from build123d import *

# Parameters (mm, degrees)
SKETCH1_R           = 1.3
SKETCH1_W           = 14
SKETCH1_H           = 14
BOSS_EXTRUDE1_DEPTH = 1


with BuildPart() as part:
    # Sketch1 → Boss-Extrude1 (new body)
    with BuildSketch(Plane(origin=(0, 0, 0), x_dir=(1, 0, 0), z_dir=(0, 1, 0))):
        with BuildLine():
            Line((27.6, 52), (-27.6, 52))
            ThreePointArc((-27.6, 52), (-28.660660172, 51.560660172), (-29.1, 50.5))
            Line((-29.1, 50.5), (-29.1, -50.5))
            ThreePointArc((-29.1, -50.5), (-28.660660172, -51.560660172), (-27.6, -52))
            Line((-27.6, -52), (27.6, -52))
            ThreePointArc((27.6, -52), (28.660660172, -51.560660172), (29.1, -50.5))
            Line((29.1, -50.5), (29.1, 50.5))
            ThreePointArc((29.1, 50.5), (28.660660172, 51.560660172), (27.6, 52))
        make_face()
        with Locations(Location((-9.525, -32.95, 0), (0, 0, 270))):
            Circle(SKETCH1_R, mode=Mode.SUBTRACT)
        with Locations(Location((9.525, -32.95, 0), (0, 0, 270))):
            Circle(SKETCH1_R, mode=Mode.SUBTRACT)
        with Locations(Location((9.525, 24.2, 0), (0, 0, 270))):
            Circle(SKETCH1_R, mode=Mode.SUBTRACT)
        with Locations(Location((-9.525, 24.2, 0), (0, 0, 270))):
            Circle(SKETCH1_R, mode=Mode.SUBTRACT)
        with Locations((0, -42.1)):
            Rectangle(SKETCH1_W, SKETCH1_H, mode=Mode.SUBTRACT)
        with Locations((19.05, -42.1)):
            Rectangle(SKETCH1_W, SKETCH1_H, mode=Mode.SUBTRACT)
        with Locations((-19.05, -42.1)):
            Rectangle(SKETCH1_W, SKETCH1_H, mode=Mode.SUBTRACT)
        with Locations((-19.05, -23.05)):
            Rectangle(SKETCH1_W, SKETCH1_H, mode=Mode.SUBTRACT)
        with Locations((0, -23.05)):
            Rectangle(SKETCH1_W, SKETCH1_H, mode=Mode.SUBTRACT)
        with Locations((19.05, -23.05)):
            Rectangle(SKETCH1_W, SKETCH1_H, mode=Mode.SUBTRACT)
        with Locations((-19.05, -4)):
            Rectangle(SKETCH1_W, SKETCH1_H, mode=Mode.SUBTRACT)
        with Locations((0, -4)):
            Rectangle(SKETCH1_W, SKETCH1_H, mode=Mode.SUBTRACT)
        with Locations((19.05, -4)):
            Rectangle(SKETCH1_W, SKETCH1_H, mode=Mode.SUBTRACT)
        with Locations((-19.05, 15.05)):
            Rectangle(SKETCH1_W, SKETCH1_H, mode=Mode.SUBTRACT)
        with Locations((0, 15.05)):
            Rectangle(SKETCH1_W, SKETCH1_H, mode=Mode.SUBTRACT)
        with Locations((19.05, 15.05)):
            Rectangle(SKETCH1_W, SKETCH1_H, mode=Mode.SUBTRACT)
    extrude(amount=BOSS_EXTRUDE1_DEPTH)


solid = part.part
The listing builds one solid part. Answer for the finished solid, in the listing's coordinates (mm). Round coordinates to 2 decimals unless told otherwise and drop trailing zeros. Write each loop counter-clockwise with the first axis right and the second up, starting at its lowest first coordinate (ties: lowest second). Pieces come first, ordered by that corner, then holes. Notation, with made-up numbers: (81, 74.5) - (89, 74.5) arc R17 ccw to (89, 104.5) - close; hole circle Ø4 at (-22, 88). An arc over 180 degrees is marked (long way). Use a Markdown table: item, result. Add a question column.
1. The part is cut by section C-C (z = 18.5). Write down the section's boundary in (x, y), and give its area (3 significant figures).
2. The part is cut by section A-A (z = -24.2). Write down the section's boundary in (x, y) (3 decimals).
3. The part is cut by section B-B (x = -25). Write down the section's boundary in (y, z).
4. The part is cut by section D-D (y = 0.6). Give the number of separate pieces and of enclosed holes in the cut face, and give its area (3 significant figures).
5. For a pull along X with two mould halves and no side action, classify faces 1 (the face through (9.58, 0.49, -25.5)), 2 (the face through (0, 0, -24)) as +X half, -X half, draft (parallel to the pull), parting line (faces both ways), or undercut.
6. A flat-ended cylindrical pin translates along its axis: P1, Ø2, axis at x = -1, z = -39.5, coming from the -Y side. Find the tip coordinate at first contact, or state that the pin passes through.
7. Consider line 1 (X direction, y = 0.2, z = 32.95) (3 decimals); line 2 (X direction, y = 0.4, z = -20.5); line 3 (Z direction, x = -3.5, y = 0.9). Determine where each line is inside the solid, lowest interval first.
Reported:
| question | item | result |
|---|---|---|
| 1 | outline | (-29.1, 0) - (-26.05, 0) - (-26.05, 1) - (-29.1, 1) - close; (-12.05, 0) - (-7, 0) - (-7, 1) - (-12.05, 1) - close; (7, 0) - (12.05, 0) - (12.05, 1) - (7, 1) - close; (26.05, 0) - (29.1, 0) - (29.1, 1) - (26.05, 1) - close |
| 1 | area | 16.2 mm^2 |
| 2 | outline | (-29.1, 0) - (-10.825, 0) - (-10.825, 1) - (-29.1, 1) - close; (-8.225, 0) - (8.225, 0) - (8.225, 1) - (-8.225, 1) - close; (10.825, 0) - (29.1, 0) - (29.1, 1) - (10.825, 1) - close |
| 3 | outline | (0, -52) - (1, -52) - (1, -22.05) - (0, -22.05) - close; (0, -8.05) - (1, -8.05) - (1, -3) - (0, -3) - close; (0, 11) - (1, 11) - (1, 16.05) - (0, 16.05) - close; (0, 30.05) - (1, 30.05) - (1, 35.1) - (0, 35.1) - close; (0, 49.1) - (1, 49.1) - (1, 52) - (0, 52) - close |
| 4 | separate pieces | 1 |
| 4 | enclosed holes | 16 |
| 4 | area | 3,680 mm^2 |
| 5 | face 1 | undercut |
| 5 | face 2 | draft |
| 6 | P1 | y = 0 |
| 7 | line 1 | -29.1 to -10.825, -8.225 to 8.225, 10.825 to 29.1 |
| 7 | line 2 | -29.1 to -26.05, -12.05 to -7, 7 to 12.05, 26.05 to 29.1 |
| 7 | line 3 | -52 to -22.05, -8.05 to -3, 11 to 16.05, 30.05 to 35.1, 49.1 to 52 |
